The model under review builds one solid part; all positions refer to its coordinate system, in mm. Coordinates: 2 decimals unless noted, no trailing zeros. Loops run counter-clockwise (first coordinate to the right, second up) from the corner with the lowest first, then second, coordinate; pieces in that order, holes last. Notation, with made-up numbers: M 8,76 L 65,76 A26 ccw 65,102 Z; hole C 89.25,-15.5 d3. An arc over 180 degrees is marked long. Write item = value, one per line. Start each with the question number.
Q1. We need section A-A on x = -75. Give the boundary of the cut face in (y, z).
Q2. Mouldability with a two-part tool opening along Y and no side actions: class faces 1 (the face through (1, -13, 3)), 2 (the face through (-9, 0, 7)), 3 (the face through (-64, 0, 3)) as released by +Y, released by -Y, zero draft, split by the parting line, or undercut.
Q3. We need section D-D on z = 13.5. Give the boundary of the cut face in (x, y), and give its area (3 significant figures).
Q4. Wall thickness on probe 1 along Y at (x, z) = (75, 20.5); probe 2 along X at (y, z) = (0.5, 26.5); probe 3 along X at (y, z) = (-2.25, 3.5): over which ranges is each line inside the solid? List them lowest first.
Q5. Clearance check with flat-ended pins moving along their axes: pin 1 Ø14.5 at (x, y) = (-23, 6) entering from +Z; pin 2 Ø7.5 at (x, z) = (1, 2) entering from -Y; pin 3 Ø5 at (y, z) = (4, 16.5) entering from -X; pin 4 Ø13 at (x, y) = (75, 0) entering from -Z. State where each tip first meets the part, or that it passes through.
Q6. We need section B-B on y = 0. Give the boundary of the cut face in (x, z).
Q7. We need section C-C on z = 4.75. Give the boundary of the cut face in (x, y).
from build123d import *

# Parameters (mm, degrees)
BOSS_EXTRUDE1_DEPTH = 7
SKETCH2_R           = 14.5
BOSS_EXTRUDE2_DEPTH = 23
SKETCH3_R           = 11
CUT_EXTRUDE1_DEPTH  = 96.501308892
CUT_EXTRUDE2_START  = -7
SKETCH4_R           = 11.1
CUT_EXTRUDE2_DEPTH  = 89.501308892


with BuildPart() as part:
    # Sketch1 → Boss-Extrude1 (new body)
    with BuildSketch(Plane.XY):
        with BuildLine():
            Line((-68.577383711, 13), (68.577383711, 13))
            ThreePointArc((68.577383711, 13), (89.5, 0), (68.577383711, -13))
            Line((68.577383711, -13), (-68.577383711, -13))
            ThreePointArc((-68.577383711, -13), (-89.5, 0), (-68.577383711, 13))
        make_face()
    extrude(amount=BOSS_EXTRUDE1_DEPTH)

    # Sketch2 → Boss-Extrude2 (add)
    with BuildSketch(Plane.XY.offset(7)):
        with Locations(Location((75, 0, 0), (0, 0, 116.291555275))):
            Circle(SKETCH2_R)
    extrude(amount=BOSS_EXTRUDE2_DEPTH)

    # Sketch3 → Cut-Extrude1 (cut, through all)
    with BuildSketch(Plane(origin=(0, 0, 0), x_dir=(-1, 0, 0), z_dir=(0, 0, -1))):
        with Locations((-75, 0)):
            Circle(SKETCH3_R)
        with Locations((75, 0)):
            Circle(SKETCH3_R)
    extrude(amount=-CUT_EXTRUDE1_DEPTH, mode=Mode.SUBTRACT)

    # Sketch4 → Cut-Extrude2 (cut, through all)
    with BuildSketch(Plane(origin=(0, 0, 0), x_dir=(-1, 0, 0), z_dir=(0, 0, -1)).offset(CUT_EXTRUDE2_START)):
        with Locations((-75, 0)):
            Circle(SKETCH4_R)
    extrude(amount=-CUT_EXTRUDE2_DEPTH, mode=Mode.SUBTRACT)


solid = part.part
Returned:
q1.outline = M -14.5,0 L -11,0 L -11,7 L -14.5,7 Z; M 11,0 L 14.5,0 L 14.5,7 L 11,7 Z
q2.face_1 = released by -Y
q2.face_2 = zero draft
q2.face_3 = undercut
q3.outline = C 75,0 d29; hole C 75,0 d22.2
q3.area = 273 mm^2
q4.probe_1 = -14.5 to -11.1, 11.1 to 14.5
q4.probe_2 = 60.51 to 63.91, 86.09 to 89.49
q4.probe_3 = -89.32 to -85.77, -64.23 to 64.23, 85.77 to 89.32
q5.pin_1 = 7
q5.pin_2 = -13
q5.pin_3 = 60.58
q5.pin_4 = through
q6.outline = M -89.5,0 L -86,0 L -86,7 L -89.5,7 Z; M -64,0 L 64,0 L 64,7 L 63.9,7 L 63.9,30 L 60.5,30 L 60.5,7 L -64,7 Z; M 86,0 L 89.5,0 L 89.5,30 L 86.1,30 L 86.1,7 L 86,7 Z
q7.outline = M -68.58,-13 L 68.58,-13 A14.5 ccw long 68.58,13 L -68.58,13 A14.5 ccw long Z; hole C -75,0 d22; hole C 75,0 d22
